Geometry: final body of the model. Coordinates: model frame, mm. A direction names the side the tool comes from. Round coordinates to 2 decimals unless told otherwise and drop trailing zeros. Loops run counter-clockwise (first coordinate to the right, second up) from the corner with the lowest first, then second, coordinate; pieces in that order, holes last. Notation, with made-up numbers: (7.5, 45) -> (62.5, 45) arc R20 ccw to (62.5, 57) -> close; hole circle Ø9 at (-27.5, -29). An arc over 180 degrees is marked (long way). Answer in a Markdown table with one row per item.
```python
from build123d import *

# Parameters (mm, degrees)
SKETCH1_W           = 47.36
SKETCH1_H           = 27.9
BOSS_EXTRUDE1_DEPTH = 5.35
SKETCH2_R           = 3.125
BOSS_EXTRUDE2_DEPTH = 6.15
SKETCH3_W           = 11.2
SKETCH3_H           = 5
CUT_EXTRUDE1_DEPTH  = 1
SKETCH5_W           = 8.9
SKETCH5_H           = 3.2
CUT_EXTRUDE2_DEPTH  = 1


with BuildPart() as part:
    # Sketch1 → Boss-Extrude1 (new, symmetric)
    with BuildSketch(Plane(origin=(0, 0, 0), x_dir=(1, 0, 0), z_dir=(0, 1, 0))):
        Rectangle(SKETCH1_W, SKETCH1_H)
    extrude(amount=BOSS_EXTRUDE1_DEPTH, both=True)

    # Sketch2 → Boss-Extrude2 (add)
    with BuildSketch(Plane(origin=(9.73, 0, -13.95), x_dir=(1, 0, 0), z_dir=(0, 0, 1))):
        with Locations((8.95, 0)):
            Circle(SKETCH2_R)
    boss_extrude2 = extrude(amount=-BOSS_EXTRUDE2_DEPTH)

    # Lustro1: Boss-Extrude2 across plane
    add(boss_extrude2.mirror(Plane.XY))

    # Sketch3 → Cut-Extrude1 (cut)
    with BuildSketch(Plane.ZY.offset(23.68)):
        with Locations((-4.65, -1.55)):
            Rectangle(SKETCH3_W, SKETCH3_H)
    extrude(amount=-CUT_EXTRUDE1_DEPTH, mode=Mode.SUBTRACT)

    # Sketch5 → Cut-Extrude2 (cut)
    with BuildSketch(Plane.ZY.offset(23.68)):
        with Locations((5.4, -0.65)):
            Rectangle(SKETCH5_W, SKETCH5_H)
    extrude(amount=-CUT_EXTRUDE2_DEPTH, mode=Mode.SUBTRACT)


solid = part.part
```
Item 1: Cut plane B-B (y = 0). Output: boundary loops of the cut face in (x, z) (3 decimals), then the cut area to 3 significant figures.
Answer:
| item | result |
|---|---|
| outline | (-23.68, -13.95) -> (15.555, -13.95) -> (15.555, -20.1) -> (21.805, -20.1) -> (21.805, -13.95) -> (23.68, -13.95) -> (23.68, 13.95) -> (21.805, 13.95) -> (21.805, 20.1) -> (15.555, 20.1) -> (15.555, 13.95) -> (-23.68, 13.95) -> (-23.68, 9.85) -> (-22.68, 9.85) -> (-22.68, -10.25) -> (-23.68, -10.25) -> close |
| area | 1,380 mm² |
Item 2: Reachability of faces 1 (the face through (21.66, 0.94, -16.98)), 2 (the face through (-23, -2, -10.25)), 3 (the face through (0, 5.35, 0)) from +Z, -Z, +X, -X, +Y, -Y: full face, straight path, thin tool, end or side. Return the list, or none.
Answer:
| item | result |
|---|---|
| face 1 | -Z |
| face 2 | -X |
| face 3 | +Z, -Z, +X, -X, +Y |
Item 3: Cut plane D-D (y = 4.5). Output: boundary loops of the cut face in (x, z), then the cut area to 3 significant figures.
Answer:
| item | result |
|---|---|
| outline | (-23.68, -13.95) -> (23.68, -13.95) -> (23.68, 13.95) -> (-23.68, 13.95) -> close |
| area | 1,320 mm² |
Item 4: Pin query (flat end, axial travel): pin 1 Ø0.5 at (x, y) = (-23, -3) entering from -Z; pin 2 Ø2.5 at (y, z) = (-2, 2) entering from -X; pin 3 Ø2 at (x, z) = (-9, -15.5) entering from +Y; pin 4 Ø4 at (x, y) = (4.5, 0.5) entering from +Z. Return the tip coordinate at first contact, or that it passes through.
Answer:
| item | result |
|---|---|
| pin 1 | stops at z = -13.95 |
| pin 2 | stops at x = -23.68 |
| pin 3 | passes through |
| pin 4 | stops at z = 13.95 |
Item 5: Cut plane A-A (x = 18.68). Output: boundary loops of the cut face in (y, z) (3 decimals).
Answer:
| item | result |
|---|---|
| outline | (-5.35, -13.95) -> (-3.125, -13.95) -> (-3.125, -20.1) -> (3.125, -20.1) -> (3.125, -13.95) -> (5.35, -13.95) -> (5.35, 13.95) -> (3.125, 13.95) -> (3.125, 20.1) -> (-3.125, 20.1) -> (-3.125, 13.95) -> (-5.35, 13.95) -> close |
Item 6: Draft query along Z for faces 4 (the face through (19, 0, -20.1)), 5 (the face through (-23, -3, 0.95)), 6 (the face through (-22.68, -1, 0)), 7 (the face through (21.66, 0.94, 16.98)). Return one class per face: pulls with the +Z half, pulls with the -Z half, needs draft (parallel to the pull), parting line crosses it, or undercut.
Answer:
| item | result |
|---|---|
| face 4 | pulls with the -Z half |
| face 5 | undercut |
| face 6 | undercut |
| face 7 | needs draft |
Item 7: Line query: probe 1 along Z at (x, y) = (-14.5, 2); probe 2 along X at (y, z) = (0.5, 5); probe 3 along X at (y, z) = (-1.25, 14). Output: solid intervals per line, ascending. Write a range as [from, to].
Answer:
| item | result |
|---|---|
| probe 1 | z = [-13.95, 13.95] |
| probe 2 | x = [-22.68, 23.68] |
| probe 3 | x = [15.82, 21.54] |
Item 8: Cut plane C-C (z = 14.5). Output: boundary loops of the cut face in (x, y) (3 decimals).
Answer:
| item | result |
|---|---|
| outline | circle Ø6.25 at (18.68, 0) |
